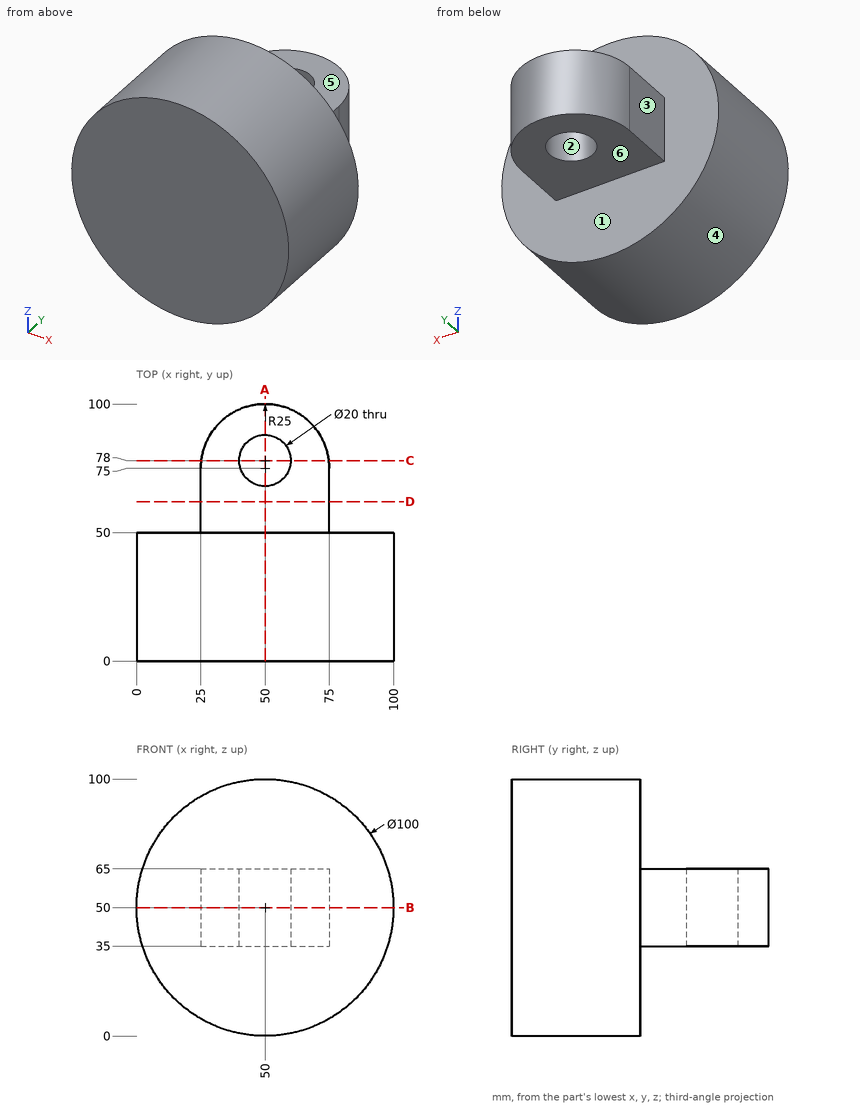
Input: dimensioned drawing with shaded views. Units: mm. Origin: part minimum x, y, z. A direction names the side the tool comes from. Coordinates: 2 decimals unless noted, no trailing zeros. Order: outer loops, then holes, each group sorted by start corner. A loop starts at its lowest first (then second) coordinate and runs counter-clockwise, first axis right, second up.
(1) Access query for the marked faces 4, 5 and 6. Directions: +Z, -Z, +X, -X, +Y, -Y. A direction counts if a zero-diameter tool reaches every point of the face in a straight line with its end or side. Return the directions, or none.
(2) Section query A-A (x = 50). Return the cut outline in (y, z).
(3) Draft query along X for the marked faces 1, 2 and 3. Return one class per face: pulls with the +X half, pulls with the -X half, needs draft (parallel to the pull), parting line crosses it, or undercut.
(4) First-contact query: pin 1 (2 mm diameter, centred on y = 76, z = 43.5, fed in from -X); pin 2 (4 mm diameter, centred on x = 62, z = 48.5, fed in from +Y); pin 3 (7.5 mm diameter, centred on y = 68, z = 46.5, fed in from +X). Flat tips, straight axial feed; report the tip coordinate or a pass-through.
(5) Section query C-C (y = 78). Return the cut outline in (x, z), plus the area to 3 significant figures.
(6) Section query B-B (z = 50). Return the cut outline in (x, y), plus the area to 3 significant figures.
(7) Material intervals for probe 1 along Y at (x, z) = (50, 55); probe 2 along Y at (x, z) = (14, 61.5); probe 3 along Y at (x, z) = (58, 53.5), sorted ascending.
(8) Section query D-D (y = 62). Return the cut outline in (x, z).
Solution:
1. face 4: +Y, -Y
1. face 5: +Z, +X, -X, +Y
1. face 6: -Z, +X, -X, +Y
2. outline: (0, 0) - (50, 0) - (50, 35) - (68, 35) - (68, 65) - (50, 65) - (50, 100) - (0, 100) - close; (88, 35) - (100, 35) - (100, 65) - (88, 65) - close
3. face 1: needs draft
3. face 2: undercut
3. face 3: pulls with the -X half
4. pin 1: stops at x = 25
4. pin 2: stops at y = 97.91
4. pin 3: stops at x = 75
5. outline: (25.18, 35) - (40, 35) - (40, 65) - (25.18, 65) - close; (60, 35) - (74.82, 35) - (74.82, 65) - (60, 65) - close
5. area: 889 mm2
6. outline: (0, 0) - (100, 0) - (100, 50) - (75, 50) - (75, 75) arc R25 ccw to (25, 75) - (25, 50) - (0, 50) - close; hole circle Ø20 at (50, 78)
6. area: 6,920 mm2
7. probe 1: y = 0 to 68, 88 to 100
7. probe 2: y = 0 to 50
7. probe 3: y = 0 to 72, 84 to 98.69
8. outline: (25, 35) - (75, 35) - (75, 65) - (25, 65) - close
